The drawing under review shows one solid part. Ordinate dimensions are in mm from its lowest x, y, z. Give positions to 0.01 mm unless a question says otherwise; leave off trailing zeros. Write each loop counter-clockwise with the first axis right and the second up, starting at its lowest first coordinate (ties: lowest second). Pieces come first, ordered by that corner, then holes. Notation, with made-up numbers: M 77,19 L 119,19 A14 cw 119,23 Z; hole C 79.5,-20 d9. An arc over 180 degrees is marked long. One line per item, written item: value. Start each with the question number.
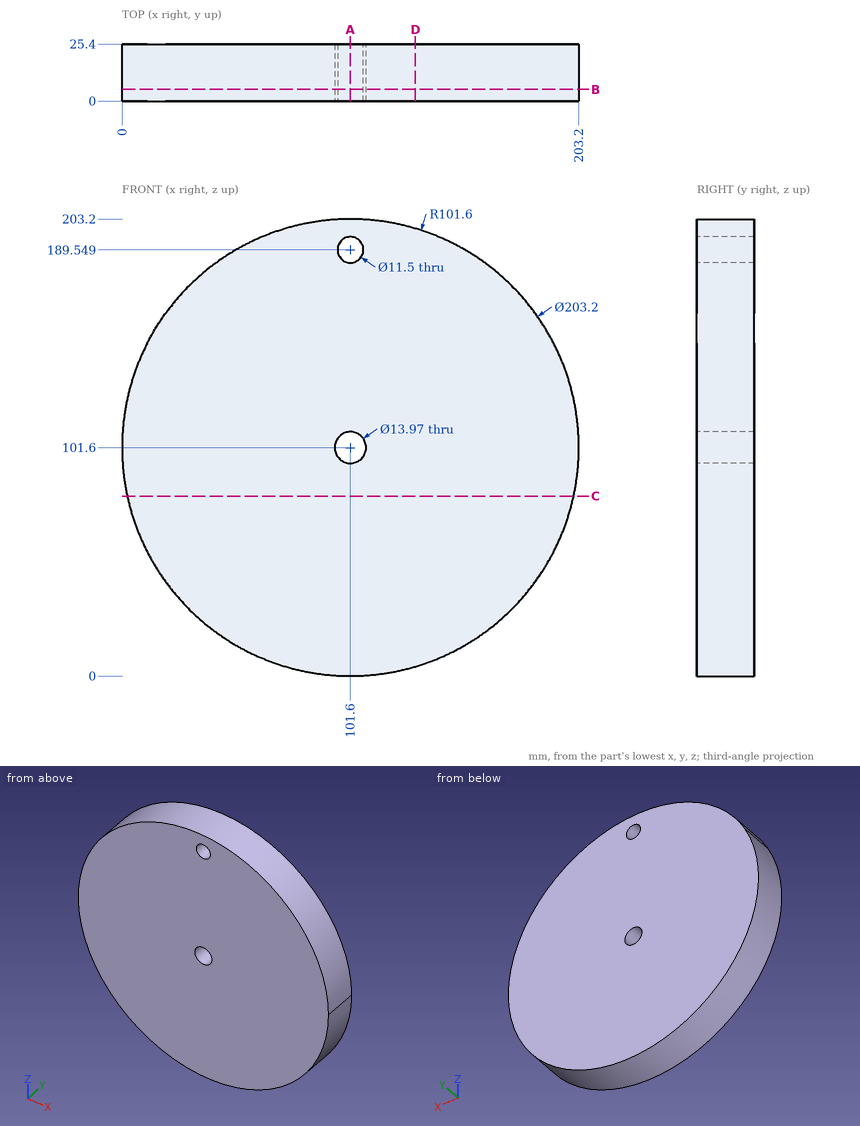
Q1. Take a section at B-B, the plane y = 5.25. State how many separate pieces and enclosed holes the cut face has, then the cut area to 3 significant figures.
Q2. Take a section at D-D, the plane x = 130.5. Give the boundary of the cut face in (y, z), then the cut area to 3 significant figures.
Q3. For P1, Ø3, axis at y = 22.5, z = 175, coming from the -X side (1 decimal); P2, Ø22.5, axis at x = 101.6, z = 101.6, coming from the -Y side; P3, Ø1.5, axis at x = 134.5, y = 14.5, coming from the -Z side; P4, Ø3, axis at y = 9.5, z = 21.5, coming from the +X side, all flat-tipped, find the tip position at first contact; note any pin that passes through.
Q4. Wall thickness on line 1 (Z direction, x = 101.6, y = 17) (1 decimal); line 2 (X direction, y = 5.25, z = 190) (1 decimal); line 3 (Z direction, x = 162.5, y = 5.5) (1 decimal): over which ranges is each line inside the solid? List them lowest first. Write a range as from..to.
Q5. Take a section at C-C, the plane z = 80. Give the boundary of the cut face in (x, y), then the cut area to 3 significant figures.
Q6. Take a section at A-A, the plane x = 101.6. Give the boundary of the cut face in (y, z) (1 decimal).
Results list:
1. separate pieces: 1
1. enclosed holes: 2
1. area: 32,200 mm^2
2. outline: M 0,4.2 L 25.4,4.2 L 25.4,199 L 0,199 Z
2. area: 4,950 mm^2
3. P1: stops at x = 29.8
3. P2: stops at y = 0
3. P3: stops at z = 5.22
3. P4: stops at x = 165.98
4. line 1: z = 0..94.6, 108.6..183.8, 195.3..203.2
4. line 2: x = 51.5..95.9, 107.3..151.7
4. line 3: z = 20.3..182.9
5. outline: M 2.32,0 L 200.88,0 L 200.88,25.4 L 2.32,25.4 Z
5. area: 5,040 mm^2
6. outline: M 0,0 L 25.4,0 L 25.4,94.6 L 0,94.6 Z; M 0,108.6 L 25.4,108.6 L 25.4,183.8 L 0,183.8 Z; M 0,195.3 L 25.4,195.3 L 25.4,203.2 L 0,203.2 Z
